CAD build for the part. Positions are in the model's coordinates, mm. A direction names the side the tool comes from. Give positions to 0.01 mm unless a question says otherwise; leave off trailing zeros. Order: outer loops, then holes, each group sorted by start corner. A loop starts at its lowest first (then second) coordinate and runs counter-clockwise, first axis right, second up. Notation, with made-up numbers: M 75.25,-12.75 L 82.25,-12.75 A13 cw 82.25,2.25 Z; hole C -11.75,73.5 d8. An arc over 180 degrees is marked long. Put each result on its own line as item: value. Start each with the question number.
1) Cut at C-C (y = 28.5). Write the cut outline in (x, z), and give its area (3 significant figures).
2) Drill centre lines: line 1 (Y direction, x = 576, z = 49.5); line 2 (Z direction, x = -49, y = 4); line 3 (Y direction, x = 224, z = 31.5). Where is each one in solid material? Low to high. Write a range as [from, to].
3) Two-plate mould, pull along X, no slides. Class faces 1 (the face through (756.41, 87.46, 42.42)), 2 (the face through (325, 76, 65)), 3 (the face through (173.98, 55.56, 32.04)): released by +X, released by -X, zero draft, split by the parting line, or undercut.
4) Cut at B-B (x = 414). Write the cut outline in (y, z), and give its area (3 significant figures).
5) Cut at A-A (z = 32.5). Write the cut outline in (x, y).
6) Pin check, flat tips, straight feed: pin 1 (4 mm diameter, centred on x = 275, z = 46, fed in from +Y); pin 2 (3 mm diameter, centred on x = 636, z = 47, fed in from -Y); pin 3 (4 mm diameter, centred on y = 79.5, z = 13.5, fed in from +X). Stop position of each tip, or through.
7) Tool access for faces 4 (the face through (-81.992, 7.395, 33.215)), 5 (the face through (568, 80, 32)), 6 (the face through (-32, 15, 32)): list every direction of +Z, -Z, +X, -X, +Y, -Y with a clear straight run to the whole face (end or side of a thin tool).
```python
from build123d import *

# Parameters (mm, degrees)
BOSS_EXTRUDE1_DEPTH = 65
FILLET1_RADIUS      = 32.5
FILLET1_LENGTH      = 15
FILLET2_RADIUS      = 32.5
FILLET2_LENGTH      = 15
SKETCH3_R           = 10
CUT_EXTRUDE1_DEPTH  = 20
SKETCH4_R           = 10
CUT_EXTRUDE2_DEPTH  = 20
SKETCH5_R           = 12.5
CUT_EXTRUDE3_DEPTH  = 20
FILLET3_R           = 5


with BuildPart() as part:
    # Sketch1 → Boss-Extrude1 (new body)
    with BuildSketch(Plane.XY):
        Polygon((-82, 0), (0, 0), (346.518069943, 80), (796.518069943, 80), (796.518069943, 95), (344.809035818, 95), (-1.709034125, 15), (-82, 15), align=None)
    extrude(amount=BOSS_EXTRUDE1_DEPTH)

    # Fillet1: full round fillet: the end face becomes a half cylinder, R = half its width
    fillet1_face = Plane((-82, 7.5, 32.5), x_dir=(0, -1, 0), z_dir=(-1, 0, 0))  # on the end face: x along it, z out of the body
    fillet1_slab = fillet1_face.offset(-FILLET1_RADIUS / 2) * Box(FILLET1_LENGTH, 2 * FILLET1_RADIUS, FILLET1_RADIUS, mode=Mode.PRIVATE)  # the body's end, R deep
    fillet1_round = Plane((-49.5, 7.5, 32.5), x_dir=(-1, 0, 0), z_dir=(0, -1, 0)) * Cylinder(FILLET1_RADIUS, FILLET1_LENGTH, mode=Mode.PRIVATE)  # its axis R under the face
    add(fillet1_slab - fillet1_round, mode=Mode.SUBTRACT)

    # Fillet2: full round fillet: the end face becomes a half cylinder, R = half its width
    fillet2_face = Plane((796.518069943, 87.5, 32.5), x_dir=(0, -1, 0), z_dir=(1, 0, 0))  # on the end face: x along it, z out of the body
    fillet2_slab = fillet2_face.offset(-FILLET2_RADIUS / 2) * Box(FILLET2_LENGTH, 2 * FILLET2_RADIUS, FILLET2_RADIUS, mode=Mode.PRIVATE)  # the body's end, R deep
    fillet2_round = Plane((764.018069943, 87.5, 32.5), x_dir=(1, 0, 0), z_dir=(0, -1, 0)) * Cylinder(FILLET2_RADIUS, FILLET2_LENGTH, mode=Mode.PRIVATE)  # its axis R under the face
    add(fillet2_slab - fillet2_round, mode=Mode.SUBTRACT)

    # Sketch3 → Cut-Extrude1 (cut)
    with BuildSketch(Plane.XZ.offset(-80)):
        with Locations(Location((466.518069943, 32.5, 0), (0, 0, 270))):
            Circle(SKETCH3_R)
    extrude(amount=-CUT_EXTRUDE1_DEPTH, mode=Mode.SUBTRACT)

    # Sketch4 → Cut-Extrude2 (cut)
    with BuildSketch(Plane.XZ):
        with Locations(Location((-49.5, 32.5, 0), (0, 0, 270))):
            Circle(SKETCH4_R)
    extrude(amount=-CUT_EXTRUDE2_DEPTH, mode=Mode.SUBTRACT)

    # Sketch5 → Cut-Extrude3 (cut)
    with BuildSketch(Plane.XZ.offset(-80)):
        with Locations(Location((764.018069943, 32.5, 0), (0, 0, 270))):
            Circle(SKETCH5_R)
    extrude(amount=-CUT_EXTRUDE3_DEPTH, mode=Mode.SUBTRACT)

    # Fillet3
    fillet3_edges = [part.edges().sort_by_distance(p)[0] for p in [
        (764.018069943, 95, 45),
        (764.018069943, 80, 45),
    ]]
    fillet(fillet3_edges, radius=FILLET3_R)


solid = part.part
```
Solution:
1. outline: M 56.77,0 L 123.45,0 L 123.45,65 L 56.77,65 Z
1. area: 4,330 mm²
2. line 1: [80, 95]
2. line 2: [0, 22.51], [42.49, 65]
2. line 3: [51.71, 67.11]
3. face 1: undercut
3. face 2: zero draft
3. face 3: released by -X
4. outline: M 80,0 L 95,0 L 95,65 L 80,65 Z
4. area: 975 mm²
5. outline: M -82,0 L -59.5,0 L -59.5,15 L -82,15 Z; M -39.5,0 L 0,0 L 346.52,80 L 456.52,80 L 456.52,95 L 344.81,95 L -1.71,15 L -39.5,15 Z; M 476.52,80 L 746.52,80 A5 ccw 751.52,85 L 751.52,90 A5 ccw 746.52,95 L 476.52,95 Z; M 776.52,85 A5 ccw 781.52,80 L 796.52,80 L 796.52,95 L 781.52,95 A5 ccw 776.52,90 Z
6. pin 1: y = 79.35
6. pin 2: y = 80
6. pin 3: x = 791.68
7. face 4: -X, +Y, -Y
7. face 5: +Z, -Z, +X, -Y
7. face 6: +Z, -Z, -X, +Y
